Part model, mm, in its own coordinate system. Face numbers are marked on the shaded views. A direction names the side the tool comes from. Coordinates: 2 decimals unless noted, no trailing zeros. Loops run counter-clockwise (first coordinate to the right, second up) from the corner with the lowest first, then second, coordinate; pieces in that order, holes last. Notation, with made-up numbers: (76, 64) - (116, 64) arc R33 cw to (116, 101) - close; hole circle Ø5 at (35.5, -11). An arc over 180 degrees is marked (long way). Use a Markdown table: item, result. Add a question column.
1. Pull direction Y, two halves, no side cores. Call the marked faces 5, 6, 7 and 8: pulls with the +Y half, pulls with the -Y half, needs draft (parallel to the pull), parting line crosses it, or undercut.
2. Band-saw the part on C-C, the plane y = -13. Give the cut face in (x, z), plus the area to 3 significant figures.
3. 3-axis set-ups, long thin cutter, end or side, ignore diameter. For the marked faces 1, 2, 3 and 4: which of +Z, -Z, +X, -X, +Y, -Y reach the whole face in a straight line?
4. Drop flat-ended pins along their axis: pin 1 (10 mm diameter, centred on y = 1.5, z = 47.5, fed in from +X); pin 2 (1 mm diameter, centred on x = -16.5, y = -22.5, fed in from -Z); pin 3 (3 mm diameter, centred on x = -29.5, z = 35.5, fed in from -Y); pin 4 (12 mm diameter, centred on x = -12, y = -40.5, fed in from -Z). Give the stop position or say it passes through.
5. Band-saw the part on A-A, the plane z = 65. Give the cut face in (x, y), plus the area to 3 significant figures.
6. Band-saw the part on B-B, the plane x = 14. Give the cut face in (y, z).
7. Band-saw the part on D-D, the plane z = 30. Give the cut face in (x, y), plus the area to 3 significant figures.
8. Wall check: probe 1 along Y at (x, z) = (10, 4); probe 2 along Z at (x, y) = (33.5, -18); probe 3 along X at (y, z) = (-5.5, 38.5). Give the ranges that are in metal, low to high. Write a range as [from, to].
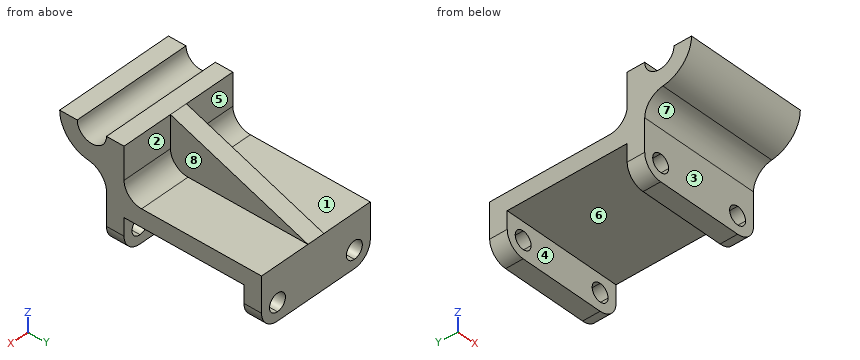
from build123d import *

# Parameters (mm, degrees)
F0_W      = 82
F0_H      = 106
F1_DEPTH  = 36
F3_R      = 12
F4_DEPTH  = 191.1
F5_R      = 12
F7_DEPTH  = 174.6
F9_W      = 82
F9_H      = 12.96312543
F10_DEPTH = 116.9
F12_DEPTH = 34
F14_DEPTH = 25
F15_W     = 12
F15_H     = 34
F16_DEPTH = 25
F18_DEPTH = 34
F19_R     = 12
F21_DEPTH = 82
F22_R     = 14


# Not quite as in the source:
# - a feature of the source that left no trace in its solid (it failed there, or was rolled back) is left out


with BuildPart() as f1:
    # F0 (on Top) → F1 (new body)
    with BuildSketch(Plane.XY):
        Rectangle(F0_W, F0_H)
    extrude(amount=F1_DEPTH)

    # F3
    f3_edges = [f1.edges().sort_by_distance(p)[0] for p in [
        (-41, 0, 0),
    ]]
    fillet(f3_edges, radius=F3_R)

    # F2 (on face) → F4 (cut)
    with BuildSketch(Plane.XZ.offset(53)):
        with BuildLine():
            ThreePointArc((-29, 18), (-35, 12), (-29, 6))
            Line((-29, 6), (-29, 12))
            Line((-29, 12), (-29, 18))
        make_face()
        with BuildLine():
            Line((-29, 12), (-29, 6))
            ThreePointArc((-29, 6), (-24.7573593129, 7.7573593129), (-23, 12))
            ThreePointArc((-23, 12), (-24.7573593129, 16.2426406871), (-29, 18))
            Line((-29, 18), (-29, 12))
        make_face()
        with BuildLine():
            Line((29, 12), (29, 6))
            ThreePointArc((29, 6), (33.2426406871, 7.7573593129), (35, 12))
            ThreePointArc((35, 12), (33.2426406871, 16.2426406871), (29, 18))
            Line((29, 18), (29, 12))
        make_face()
        with BuildLine():
            ThreePointArc((29, 18), (23, 12), (29, 6))
            Line((29, 6), (29, 12))
            Line((29, 12), (29, 18))
        make_face()
    extrude(amount=-F4_DEPTH, mode=Mode.SUBTRACT)

    # F5
    f5_edges = [f1.edges().sort_by_distance(p)[0] for p in [
        (41, 0, 0),
    ]]
    fillet(f5_edges, radius=F5_R)

    # F6 (on face) → F7 (cut)
    with BuildSketch(Plane.YZ.offset(41)):
        Polygon((41, 24), (-30.1027745008, 24), (-41, 24), (-41, 12), (41, 12), align=None)
    extrude(amount=-F7_DEPTH, mode=Mode.SUBTRACT)

    # F9 (on face) → F10 (cut)
    with BuildSketch(Plane.YZ.offset(41)):
        with Locations((0, 5.518437285)):
            Rectangle(F9_W, F9_H)
    extrude(amount=-F10_DEPTH, mode=Mode.SUBTRACT)

    # F11 (on face) → F12 (join)
    with BuildSketch(Plane.XY.offset(36)):
        Polygon((0, 53), (-6, 53), (-6, -53), (6, -53), (6, 53), align=None)
    extrude(amount=F12_DEPTH)

    # F13 (on face) → F14 (cut)
    with BuildSketch(Plane(origin=(-6, 0, 0), x_dir=(0, -1, 0), z_dir=(-1, 0, 0))):
        Polygon((-53, 70), (-53, 36), (41, 70), align=None)
    extrude(amount=-F14_DEPTH, mode=Mode.SUBTRACT)

    # F15 (on face) → F16 (cut)
    with BuildSketch(Plane(origin=(-6, 0, 0), x_dir=(0, -1, 0), z_dir=(-1, 0, 0))):
        with Locations((47, 53)):
            Rectangle(F15_W, F15_H)
    extrude(amount=-F16_DEPTH, mode=Mode.SUBTRACT)

    # F17 (on face) → F18 (join)
    with BuildSketch(Plane.XY.offset(36)):
        Polygon((41, -53), (41, -41), (6, -41), (-6, -41), (-41, -41), (-41, -53), align=None)
    extrude(amount=F18_DEPTH)

    # F19
    f19_edges = [f1.edges().sort_by_distance(p)[0] for p in [
        (-23.5, -41, 36),
        (23.5, -41, 36),
    ]]
    fillet(f19_edges, radius=F19_R)

    # F20 (on face) → F21 (join, through all)
    with BuildSketch(Plane(origin=(-41, 0, 0), x_dir=(0, -1, 0), z_dir=(-1, 0, 0))):
        with BuildLine():
            Line((53, 70), (53, 50.4040820577))
            ThreePointArc((53, 50.4040820577), (74.4891252931, 51.2383369607), (85, 70))
            Line((85, 70), (73, 70))
            ThreePointArc((73, 70), (63, 60), (53, 70))
        make_face()
        with BuildLine():
            Line((53, 70), (41, 70))
            ThreePointArc((41, 70), (44.2383369607, 58.5108747069), (53, 50.4040820577))
            Line((53, 50.4040820577), (53, 70))
        make_face()
    extrude(amount=-F21_DEPTH)

    # F22
    f22_edges = [f1.edges().sort_by_distance(p)[0] for p in [
        (0, -53, 50.404082),
    ]]
    fillet(f22_edges, radius=F22_R)


solid = f1.part
Geometry check:
| question | item | result |
|---|---|---|
| 1 | face 5 | pulls with the +Y half |
| 1 | face 6 | undercut |
| 1 | face 7 | pulls with the -Y half |
| 1 | face 8 | needs draft |
| 2 | outline | (-41, 24) - (41, 24) - (41, 36) - (6, 36) - (6, 59.87) - (-6, 59.87) - (-6, 36) - (-41, 36) - close |
| 2 | area | 1,270 mm^2 |
| 3 | face 1 | +Z, -X, +Y |
| 3 | face 2 | +Z, +X, +Y |
| 3 | face 3 | -Z, +X, -X, -Y |
| 3 | face 4 | -Z, +X, -X |
| 4 | pin 1 | stops at x = 6 |
| 4 | pin 2 | stops at z = 24 |
| 4 | pin 3 | stops at y = -53.28 |
| 4 | pin 4 | stops at z = 0 |
| 5 | outline | (-41, -84.42) - (41, -84.42) - (41, -71.66) - (-41, -71.66) - close; (-41, -54.34) - (41, -54.34) - (41, -41) - (6, -41) - (6, -27.18) - (-6, -27.18) - (-6, -41) - (-41, -41) - close |
| 5 | area | 2,310 mm^2 |
| 6 | outline | (-85, 70) arc R22 ccw to (-65.44, 48.14) arc R14 cw to (-53, 34.22) - (-53, 0) - (-41, 0) - (-41, 24) - (41, 24) - (41, 0) - (53, 0) - (53, 36) - (-29, 36) arc R12 cw to (-41, 48) - (-41, 70) - (-53, 70) arc R10 cw to (-73, 70) - close |
| 7 | outline | (-41, -53) - (41, -53) - (41, 53) - (-41, 53) - close |
| 7 | area | 8,690 mm^2 |
| 8 | probe 1 | y = [-53, -41], [41, 53] |
| 8 | probe 2 | z = [24, 36] |
| 8 | probe 3 | x = [-6, 6] |
